Geometry: final body of the model. Coordinates: model frame, mm. A direction names the side the tool comes from. Coordinates: 2 decimals unless noted, no trailing zeros. Loops run counter-clockwise (first coordinate to the right, second up) from the corner with the lowest first, then second, coordinate; pieces in that order, holes last. Notation, with made-up numbers: (65.5, 45) -> (104.5, 45) arc R31 ccw to (104.5, 70) -> close; hole circle Ø2 at (77, 76). An arc over 180 degrees is marked (long way). One line per item, written item: value. Start each with the question number.
from build123d import *

# Parameters (mm, degrees)
SKETCH1_W                                     = 13
SKETCH1_H                                     = 25
SKETCH1_R                                     = 2
BOSS_EXTRUDE1_DEPTH                           = 8
SKETCH2_W                                     = 13
SKETCH2_H                                     = 32
SKETCH2_R                                     = 2
BOSS_EXTRUDE2_DEPTH                           = 6
CSK_FOR_M4_COUNTERSUNK_FLAT_HEAD1_D           = 4.5
CSK_FOR_M4_COUNTERSUNK_FLAT_HEAD1_CSINK_D     = 9.4
CSK_FOR_M4_COUNTERSUNK_FLAT_HEAD1_CSINK_ANGLE = 90


with BuildPart() as part:
    # Sketch1 → Boss-Extrude1 (new body)
    with BuildSketch(Plane.XY):
        Rectangle(SKETCH1_W, SKETCH1_H)
        with Locations((0, -7.5)):
            Circle(SKETCH1_R, mode=Mode.SUBTRACT)
        with Locations(Location((0, 7.5, 0), (0, 0, 180))):
            Circle(SKETCH1_R, mode=Mode.SUBTRACT)
    extrude(amount=BOSS_EXTRUDE1_DEPTH)

    # Sketch2 → Boss-Extrude2 (add)
    with BuildSketch(Plane(origin=(0, 0, 0), x_dir=(-1, 0, 0), z_dir=(0, 0, -1))):
        with Locations((0, 28.5)):
            Rectangle(SKETCH2_W, SKETCH2_H)
        with Locations((0, 39.5)):
            Circle(SKETCH2_R, mode=Mode.SUBTRACT)
        with Locations((0, 19.5)):
            Circle(SKETCH2_R, mode=Mode.SUBTRACT)
    extrude(amount=-BOSS_EXTRUDE2_DEPTH)

    # CSK for M4 Countersunk Flat Head1 (through all)
    with Locations(Plane(origin=(0, 0, 0), x_dir=(-1, 0, 0), z_dir=(0, 0, -1))):
        with Locations((0, -7.5), (0, 7.5)):
            CounterSinkHole(CSK_FOR_M4_COUNTERSUNK_FLAT_HEAD1_D / 2, CSK_FOR_M4_COUNTERSUNK_FLAT_HEAD1_CSINK_D / 2, counter_sink_angle=CSK_FOR_M4_COUNTERSUNK_FLAT_HEAD1_CSINK_ANGLE)


solid = part.part
1. Section A-A on y = 19.5. Return the cut outline in (x, z), plus the area to 3 significant figures.
2. Set-up query: faces 1 (the face through (0, 23, 0)), 2 (the face through (0, 29, 6)). Return all of +Z, -Z, +X, -X, +Y, -Y with unobstructed straight access to the full face (end or side cutting, diameter ignored); none if empty.
3. Pin query (flat end, axial travel): pin 1 Ø6.5 at (x, y) = (-1.5, 26) entering from +Z; pin 2 Ø1.6 at (x, z) = (-2, 6.5) entering from +Y; pin 3 Ø1 at (x, z) = (-4, 7) entering from +Y. Return the tip coordinate at first contact, or that it passes through.
4. Section B-B on x = 0. Return the cut outline in (y, z).
5. Line query: L1, parallel to Y at x = 0, z = 5.25; L2, parallel to X at y = -7.5, z = 5.15; L3, parallel to Y at x = -0.75, z = 4.25. Output: solid intervals per line, ascending. Write a range as [from, to].
6. Section D-D on y = -7.5. Return the cut outline in (x, z), plus the area to 3 significant figures.
7. Draft query along Y for faces 3 (the face through (0, 12.5, 7)), 4 (the face through (0, -12.5, 4)), 5 (the face through (0.434, 37.548, 2.958)). Return one class per face: released by +Y, released by -Y, zero draft, split by the parting line, or undercut.
8. Section C-C on z = 1.25. Return the cut outline in (x, y), plus the area to 3 significant figures.
Checks:
1. outline: (-6.5, 0) -> (-2, 0) -> (-2, 6) -> (-6.5, 6) -> close; (2, 0) -> (6.5, 0) -> (6.5, 6) -> (2, 6) -> close
1. area: 54.0 mm²
2. face 1: -Z, +X, -X, +Y, -Y
2. face 2: +Z, +X, -X, +Y
3. pin 1: z = 6
3. pin 2: y = 44.5
3. pin 3: y = 12.5
4. outline: (-12.5, 0) -> (-12.2, 0) -> (-9.75, 2.45) -> (-9.75, 8) -> (-12.5, 8) -> close; (-5.25, 2.45) -> (-2.8, 0) -> (2.8, 0) -> (5.25, 2.45) -> (5.25, 8) -> (-5.25, 8) -> close; (9.75, 2.45) -> (12.2, 0) -> (17.5, 0) -> (17.5, 6) -> (12.5, 6) -> (12.5, 8) -> (9.75, 8) -> close; (21.5, 0) -> (37.5, 0) -> (37.5, 6) -> (21.5, 6) -> close; (41.5, 0) -> (44.5, 0) -> (44.5, 6) -> (41.5, 6) -> close
5. L1: [-12.5, -9.75], [-5.25, 5.25], [9.75, 17.5], [21.5, 37.5], [41.5, 44.5]
5. L2: [-6.5, -2.25], [2.25, 6.5]
5. L3: [-12.5, -9.62], [-5.38, 5.38], [9.62, 17.65], [21.35, 37.65], [41.35, 44.5]
6. outline: (-6.5, 0) -> (-4.7, 0) -> (-2.25, 2.45) -> (-2.25, 8) -> (-6.5, 8) -> close; (2.25, 2.45) -> (4.7, 0) -> (6.5, 0) -> (6.5, 8) -> (2.25, 8) -> close
6. area: 62.0 mm²
7. face 3: released by +Y
7. face 4: released by -Y
7. face 5: undercut
8. outline: (-6.5, -12.5) -> (6.5, -12.5) -> (6.5, 44.5) -> (-6.5, 44.5) -> close; hole circle Ø6.9 at (0, -7.5); hole circle Ø6.9 at (0, 7.5); hole circle Ø4 at (0, 19.5); hole circle Ø4 at (0, 39.5)
8. area: 641 mm²
